The listing builds one solid part. Answer for the finished solid, in the listing's coordinates (mm). A direction names the side the tool comes from. Coordinates: 2 decimals unless noted, no trailing zeros. Loops run counter-clockwise (first coordinate to the right, second up) from the corner with the lowest first, then second, coordinate; pieces in that order, holes last. Notation, with made-up numbers: M -27.75,-28.5 L -8.75,-28.5 A12 cw -8.75,-8.5 Z; hole C -38,5.5 d10. An arc over 180 degrees is marked long. Return JSON: item names as keys, results as strings. Group by question number.
1. Which of the six approach directions +Z, -Z, +X, -X, +Y, -Y give full straight-line access (tool end or side, diameter ignored) to faces 4 (the face through (24, 2, 5)), 5 (the face through (36.876, 1, 3)), 6 (the face through (25.64, 1.01, 0.74))?
2. Straight lines are drawn through the part: L1, parallel to X at y = 7.75, z = 3.5; L2, parallel to Y at x = 44, z = 7.75; L3, parallel to Y at x = 41, z = 9.25. For each, find the intervals that lie inside material, in ascending order. Write a range as from..to.
3. Section C-C (x = 43.5) is taken. Write down the section's boundary in (y, z), then the cut area to 3 significant figures.
4. Given P1, Ø1, axis at y = 3.5, z = 6.5, coming from the -X side; P2, Ø4, axis at y = 3, z = 5, coming from the -X side, each flat-ended and moving along its own axis, determine where each tip first touches the part or whether it passes through.
5. Section D-D (y = 7.25) is taken. Write down the section's boundary in (x, z).
6. Section B-B (y = 1) is taken. Write down the section's boundary in (x, z).
7. Section A-A (z = 7.5) is taken. Write down the section's boundary in (x, y), then the cut area to 3 significant figures.
8. The mould has two halves that part along X. Classify faces 1 (the face through (50, 5, 9.709)), 2 (the face through (36.21, 1.01, 1.55)), 3 (the face through (49, 5, 5)): pulls with the +X half, pulls with the -X half, needs draft (parallel to the pull), parting line crosses it, or undercut.
```python
from build123d import *

# Parameters (mm, degrees)
SKETCH_1_W               = 52
SKETCH_1_H               = 10
EXTRUDE_1_DEPTH          = 2
SKETCH_5_R               = 0.6
CUT_EXTRUDE_1_DEPTH      = 53.990565198
SKETCH_6_W               = 3
SKETCH_6_H               = 10
EXTRUDE_2_DEPTH          = 6
CUT_EXTRUDE_2_DEPTH      = 54.291650378
CUT_EXTRUDE_3_DEPTH      = 54.553711356
CUT_EXTRUDE_3_DEPTH_BACK = 54.553711356


with BuildPart() as part:
    # 草图1 → 凸台-拉伸1 (new body)
    with BuildSketch(Plane(origin=(0, 0, 0), x_dir=(1, 0, 0), z_dir=(0, 1, 0))):
        with Locations((26, -5)):
            Rectangle(SKETCH_1_W, SKETCH_1_H)
    extrude(amount=EXTRUDE_1_DEPTH)

    # 草图5 → 切除-拉伸1 (cut, through all)
    with BuildSketch(Plane(origin=(0, 2, 0), x_dir=(1, 0, 0), z_dir=(0, 1, 0))):
        with Locations(Location((36.226363192, -2.7, 0), (0, 0, 270))):
            Circle(SKETCH_5_R)
        with Locations(Location((10.926363192, -2.7, 0), (0, 0, 270))):
            Circle(SKETCH_5_R)
    extrude(amount=-CUT_EXTRUDE_1_DEPTH, mode=Mode.SUBTRACT)

    # 草图6 → 凸台-拉伸2 (add)
    with BuildSketch(Plane(origin=(0, 2, 0), x_dir=(1, 0, 0), z_dir=(0, 1, 0))):
        with Locations((50.5, -5)):
            Rectangle(SKETCH_6_W, SKETCH_6_H)
    extrude(amount=EXTRUDE_2_DEPTH)

    # 草图7 → 切除-拉伸2 (cut, through all)
    with BuildSketch(Plane(origin=(0, 2, 0), x_dir=(1, 0, 0), z_dir=(0, 1, 0))):
        with BuildLine():
            Line((11.626363192, -2.2), (11.626363192, -3.2))
            ThreePointArc((11.626363192, -3.2), (10.926363192, -3.9), (10.226363192, -3.2))
            Line((10.226363192, -3.2), (10.226363192, -2.2))
            ThreePointArc((10.226363192, -2.2), (10.926363192, -1.5), (11.626363192, -2.2))
        make_face()
        with BuildLine():
            Line((36.876363192, -2.2), (36.876363192, -3.2))
            ThreePointArc((36.876363192, -3.2), (36.226363192, -3.85), (35.576363192, -3.2))
            Line((35.576363192, -3.2), (35.576363192, -2.2))
            ThreePointArc((35.576363192, -2.2), (36.226363192, -1.55), (36.876363192, -2.2))
        make_face()
    extrude(amount=-CUT_EXTRUDE_2_DEPTH, mode=Mode.SUBTRACT)

    # 草图9 → 切除-拉伸3 (cut, two sides: drawn at the far end of the back side and taken through both)
    with BuildSketch(Plane(origin=(52, 0, 0), x_dir=(0, 0, -1), z_dir=(1, 0, 0)).offset(-CUT_EXTRUDE_3_DEPTH_BACK)):
        Polygon((-0.290909091, 2), (-1.2, 0), (0, 0), (0, 8), (-0.290909091, 8), align=None)
        Polygon((-9.709090909, 2), (-8.8, 0), (-10, 0), (-10, 8), (-9.709090909, 8), align=None)
    extrude(amount=CUT_EXTRUDE_3_DEPTH + CUT_EXTRUDE_3_DEPTH_BACK, mode=Mode.SUBTRACT)


solid = part.part
```
Worked out:
{
 "1": {"face 4": "+Z, -Z, -X, +Y", "face 5": "+Y, -Y", "face 6": "-Z, +X, -X, -Y"},
 "2": {"L1": "49..52", "L2": "0..2", "L3": "0.99..2"},
 "3": {"outline": "M 0,1.2 L 2,0.29 L 2,9.71 L 0,8.8 Z", "area": "17.0 mm^2"},
 "4": {"P1": "x = 49", "P2": "x = 0"},
 "5": {"outline": "M 49,0.29 L 52,0.29 L 52,9.71 L 49,9.71 Z"},
 "6": {"outline": "M 0,0.75 L 52,0.75 L 52,9.25 L 0,9.25 Z; hole M 10.23,2.2 A0.7 ccw 11.63,2.2 L 11.63,3.2 A0.7 ccw 10.23,3.2 Z; hole M 35.58,2.2 A0.65 ccw 36.88,2.2 L 36.88,3.2 A0.65 ccw 35.58,3.2 Z"},
 "7": {"outline": "M 0,0 L 52,0 L 52,8 L 49,8 L 49,2 L 0,2 Z", "area": "122 mm^2"},
 "8": {"face 1": "needs draft", "face 2": "undercut", "face 3": "pulls with the -X half"}
}
